from build123d import *

# Parameters (mm, degrees)
F1_DEPTH = 2
F2_R     = 10
F3_DEPTH = 2
F4_R     = 2.5
F5_DEPTH = 2


with BuildPart() as f1:
    # F0 (on Top) → F1 (new body)
    with BuildSketch(Plane.XY):
        with BuildLine():
            ThreePointArc((-4.993837, 19.290927), (-7.402673, 13.475481), (-13.643415, 14.297091))
            ThreePointArc((-13.643415, 14.297091), (-21.776508, 13.226349), (-18.637252, 5.647512))
            ThreePointArc((-18.637252, 5.647512), (-14.805346, 0.653676), (-18.637252, -4.340161))
            ThreePointArc((-18.637252, -4.340161), (-21.776508, -11.918997), (-13.643415, -12.989739))
            ThreePointArc((-13.643415, -12.989739), (-7.402673, -12.16813), (-4.993837, -17.983576))
            ThreePointArc((-4.993837, -17.983576), (0, -24.49167), (4.993837, -17.983576))
            ThreePointArc((4.993837, -17.983576), (7.402673, -12.16813), (13.643415, -12.989739))
            ThreePointArc((13.643415, -12.989739), (21.776508, -11.918997), (18.637252, -4.340161))
            ThreePointArc((18.637252, -4.340161), (14.805346, 0.653676), (18.637252, 5.647512))
            ThreePointArc((18.637252, 5.647512), (21.776508, 13.226349), (13.643415, 14.297091))
            ThreePointArc((13.643415, 14.297091), (7.402673, 13.475481), (4.993837, 19.290927))
            ThreePointArc((4.993837, 19.290927), (0, 25.799022), (-4.993837, 19.290927))
        make_face()
    extrude(amount=F1_DEPTH)

    # F2 (on face) → F3 (join)
    with BuildSketch(Plane.XY.offset(2)):
        Circle(F2_R)
    extrude(amount=F3_DEPTH)

    # F4 (on face) → F5 (join)
    with BuildSketch(Plane.XY.offset(4)):
        with BuildLine():
            Line((-5, 0), (0, 0))
            Line((0, 0), (5, 0))
            Line((5, 0), (5, 40))
            ThreePointArc((5, 40), (0, 45), (-5, 40))
            Line((-5, 40), (-5, 0))
        make_face()
        with Locations((0, 40)):
            Circle(F4_R, mode=Mode.SUBTRACT)
    extrude(amount=-F5_DEPTH)


solid = f1.part
Design review of the part built by this model. Coordinates are the model's own, in mm. A direction names the side the tool comes from. Give positions to 0.01 mm unless a question says otherwise; leave off trailing zeros. Order: outer loops, then holes, each group sorted by start corner. A loop starts at its lowest first (then second) coordinate and runs counter-clockwise, first axis right, second up.
1. To check wall thickness, follow L1, parallel to Y at x = 0, z = 3.1; L2, parallel to X at y = 16.5, z = 3.8; L3, parallel to Y at x = 10, z = 0.55. State the ranges of each line that lie inside material, in increasing order.
Solution:
L1: y = -10 to 37.5, 42.5 to 45
L2: x = -5 to 5
L3: y = -11.48 to 12.78
2. Add section D-D, the plane x = -15.5. State the section outline as (y, z) points, then the cut area to 3 significant figures.
Solution:
outline: (-14.18, 0) - (-1.93, 0) - (-1.93, 2) - (-14.18, 2) - close; (3.24, 0) - (15.49, 0) - (15.49, 2) - (3.24, 2) - close
area: 49.0 mm2
3. Add section A-A, the plane x = 0. State the section outline as (y, z) points, then the cut area to 3 significant figures.
Solution:
outline: (-24.49, 0) - (25.8, 0) - (25.8, 2) - (37.5, 2) - (37.5, 4) - (-10, 4) - (-10, 2) - (-24.49, 2) - close; (42.5, 2) - (45, 2) - (45, 4) - (42.5, 4) - close
area: 201 mm2
4. Add section C-C, the plane y = 0. State the section outline as (x, z) points.
Solution:
outline: (-14.85, 0) - (14.85, 0) - (14.85, 2) - (10, 2) - (10, 4) - (-10, 4) - (-10, 2) - (-14.85, 2) - close
5. For pin 1 Ø11 at (x, y) = (1.5, 34.5) entering from -Z; pin 2 Ø1.5 at (x, y) = (-7, 32) entering from -Z; pin 3 Ø1.6 at (y, z) = (20, 3) entering from +X; pin 4 Ø1.6 at (y, z) = (26, 3.5) entering from -X, all flat-tipped, find the tip position at first contact; note any pin that passes through.
Solution:
pin 1: stops at z = 2
pin 2: passes through
pin 3: stops at x = 5
pin 4: stops at x = -5
6. Tool access review of faces 1 (the flat face through (0, 1, 0)), 2 (the flat face through (-5, 25, 3)), 3 (the flat face through (5, 24, 3)), 4 (the flat face through (0, 12, 4)), 5 (the cylindrical face through (0, -10, 3)): name each direction out of +Z, -Z, +X, -X, +Y, -Y from which nothing blocks a thin tool from reaching the whole face with its end or side.
Solution:
face 1: -Z, +X, -X, +Y, -Y
face 2: +Z, -X, +Y
face 3: +Z, +X, +Y
face 4: +Z, +X, -X, +Y, -Y
face 5: +Z
7. Add section B-B, the plane z = 3.4. State the section outline as (x, y) points.
Solution:
outline: (-5, 8.66) arc R10 ccw (long way) to (5, 8.66) - (5, 40) arc R5 ccw to (-5, 40) - close; hole circle Ø5 at (0, 40)
